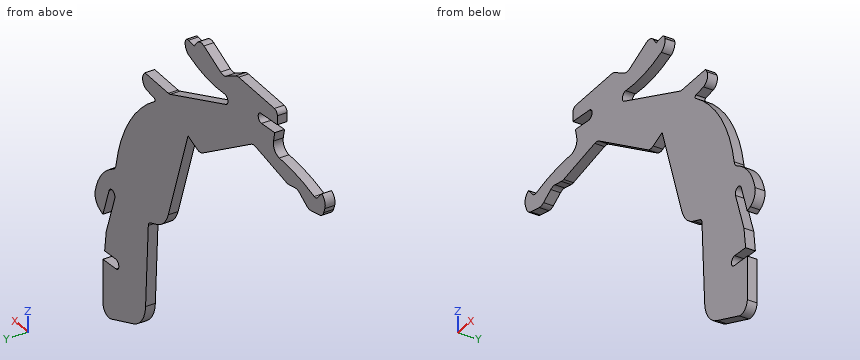
```python
from build123d import *

# Parameters (mm, degrees)
BOSS_EXTRUDE1_DEPTH = 3
FILLET1_R           = 3
FILLET2_R           = 1.5
FILLET3_R           = 10
FILLET4_R           = 3
FILLET5_R           = 4
FILLET6_R           = 2.5
FILLET7_R           = 0.5


with BuildPart() as part:
    # Sketch3 → Boss-Extrude1 (new body)
    with BuildSketch(Plane(origin=(0, 0, 0), x_dir=(1, 0, 0), z_dir=(0, 1, 0))):
        with BuildLine():
            Line((7.923093171, 8.181542538), (1.28839884, 7.442154357))
            Line((1.28839884, 7.442154357), (2.76822933, 14.19))
            ThreePointArc((2.76822933, 14.19), (-8.413807268, 14.494015924), (-19.359710867, 16.8))
            Line((-19.359710867, 16.8), (-22.216794933, 13.666296862))
            Line((-22.216794933, 13.666296862), (-24.820279869, 14.62298821))
            Line((-24.820279869, 14.62298821), (-22.646481841, 20.53863742))
            Line((-22.646481841, 20.53863742), (-15.703804617, 22.111794774))
            Line((-15.703804617, 22.111794774), (-10.073302156, 18.818482014))
            Line((-10.073302156, 18.818482014), (-5.186450964, 19.880840969))
            Line((-5.186450964, 19.880840969), (12.13, 16.8))
            Line((12.13, 16.8), (38.76, 34.29))
            Line((38.76, 34.29), (44.7, 32))
            Line((44.7, 32), (56.058554748, 66.4069852))
            Line((56.058554748, 66.4069852), (64.552315124, 69.756868371))
            Line((64.552315124, 69.756868371), (66.29, 103.00790875))
            Line((66.29, 103.00790875), (87.31, 111.63))
            Line((87.31, 111.63), (87.31, 93.591357519))
            Line((87.31, 93.591357519), (80.722672152, 93.01504101))
            ThreePointArc((80.722672152, 93.01504101), (79.359113719, 91.390015348), (80.984139381, 90.026456915))
            Line((80.984139381, 90.026456915), (86.46321022, 90.505813501))
            Line((86.46321022, 90.505813501), (85.632866314, 84))
            Line((85.632866314, 84), (81.389705108, 71.508585308))
            ThreePointArc((81.389705108, 71.508585308), (82.327545423, 69.605835839), (84.230294892, 70.543676154))
            Line((84.230294892, 70.543676154), (87.31, 79.61))
            Line((87.31, 79.61), (91.618486592, 77.887634392))
            ThreePointArc((91.618486592, 77.887634392), (88.600013238, 68.48894743), (80.984139381, 62.208424889))
            ThreePointArc((80.984139381, 62.208424889), (74.158506271, 43.709858628), (60.297831214, 29.686025056))
            Line((60.297831214, 29.686025056), (68.03871852, 28.66301442))
            ThreePointArc((68.03871852, 28.66301442), (67.586257486, 26.243028794), (66.29, 24.15))
            Line((66.29, 24.15), (54.05, 24.15))
            Line((54.05, 24.15), (25.830040494, 11.99))
            ThreePointArc((25.830040494, 11.99), (24.800734775, 10.253880031), (26.431506195, 9.064692331))
            ThreePointArc((26.431506195, 9.064692331), (36.664028635, 8.803570476), (46.46571567, 5.854056721))
            Line((46.46571567, 5.854056721), (45.9, 1.991540554))
            Line((45.9, 1.991540554), (41.660045255, 2.482673431))
            Line((41.660045255, 2.482673431), (38.9, -1.2))
            Line((38.9, -1.2), (27.015518097, 3.924692331))
            Line((27.015518097, 3.924692331), (20.16, 0))
            Line((20.16, 0), (0, 0))
            Line((0, 0), (0, 4.28))
            Line((0, 4.28), (8.255364291, 5.2))
            ThreePointArc((8.255364291, 5.2), (9.58, 6.856906829), (7.923093171, 8.181542538))
        make_face()
    extrude(amount=BOSS_EXTRUDE1_DEPTH)

    # Fillet1
    # the kernel refuses this fillet: 3 mm, written as the material it adds along each edge
    with BuildSketch(Plane(origin=(80.984139381, 0, -62.208424889), x_dir=(0.9022478681487618, 0, -0.4312177923289046), z_dir=(0, 1, 0))) as fillet1_piece_1:
        with BuildLine():
            CenterArc((1.578679862, -2.997421373), FILLET1_R, 92.37575888, 52.157589609)
            ThreePointArc((-0.864680258, -1.256734347), (-0.427200708, -0.631903288), (0, 0))
            ThreePointArc((0, 0), (0.72716053, -0.015077949), (1.45432106, 0))
        make_face()
    extrude(amount=3)
    with BuildSketch(Plane(origin=(27.015518097, 0, -3.924692331), x_dir=(0.9182659150547935, 0, 0.39596427774305953), z_dir=(0, 1, 0))) as fillet1_piece_2:
        with BuildLine():
            CenterArc((FILLET1_R * 0.49985366711, -FILLET1_R), FILLET1_R, 90, 53.116686758)
            Line((-FILLET1_R * 0.300005823165, -FILLET1_R * 0.399812699386), (0, 0))
            Line((0, 0), (FILLET1_R * 0.49985366711, 0))
        make_face()
    extrude(amount=3)
    with BuildSketch(Plane(origin=(12.13, 0, -16.8), x_dir=(-0.9845393680489544, 0, -0.17516344584919966), z_dir=(0, 1, 0))) as fillet1_piece_3:
        with BuildLine():
            CenterArc((FILLET1_R * 0.397788634748, -FILLET1_R), FILLET1_R, 90, 43.384200988)
            Line((-FILLET1_R * 0.289098500769, -FILLET1_R * 0.273235895863), (0, 0))
            Line((0, 0), (FILLET1_R * 0.397788634748, 0))
        make_face()
    extrude(amount=3)
    with BuildSketch(Plane(origin=(-10.073302156, 0, -18.818482014), x_dir=(-0.863187603129405, 0, -0.5048833150379528), z_dir=(0, 1, 0))) as fillet1_piece_4:
        with BuildLine():
            CenterArc((FILLET1_R * 0.389766900576, -FILLET1_R), FILLET1_R, 90, 42.58838059)
            Line((-FILLET1_R * 0.286959776942, -FILLET1_R * 0.263765659633), (0, 0))
            Line((0, 0), (FILLET1_R * 0.389766900576, 0))
        make_face()
    extrude(amount=3)
    with BuildSketch(Plane(origin=(2.76822933, 0, -14.19), x_dir=(-0.21421340809022724, 0, 0.9767868835085624), z_dir=(0, 1, 0))) as fillet1_piece_5:
        with BuildLine():
            CenterArc((3.855271405, -3), FILLET1_R, 90, 102.505548925)
            ThreePointArc((0.926446282, -3.649602493), (0.490902504, -1.81777488), (0, 0))
            Line((0, 0), (3.855271405, 0))
        make_face()
    extrude(amount=3)
    # the kernel refuses this fillet: 3 mm, written as the material it takes off along each edge
    with BuildSketch(Plane(origin=(-24.820279869, -7.478630688, -14.62298821), x_dir=(0.9386336815677853, 0, 0.3449156590044952), z_dir=(0, 1, 0))) as fillet1_2_piece_1:
        with BuildLine():
            CenterArc((3, 2.991452275), FILLET1_R, 180, 85.673811508)
            Line((0, 2.991452275), (0, 0))
            Line((0, 0), (2.773696477, 0))
        make_face()
    extrude(amount=17.957261376, mode=Mode.SUBTRACT)
    with BuildSketch(Plane(origin=(20.16, -1.994934097, 0), x_dir=(0.8678473261649016, 0, -0.4968309757537575), z_dir=(0, 1, 0))) as fillet1_2_piece_2:
        with BuildLine():
            CenterArc((FILLET1_R * 0.265991212876, FILLET1_R), FILLET1_R, 240.209440415, 29.790559585)
            Line((-FILLET1_R * 0.230839762878, FILLET1_R * 0.132152673835), (0, 0))
            Line((0, 0), (FILLET1_R * 0.265991212876, 0))
        make_face()
    extrude(amount=6.989868193, mode=Mode.SUBTRACT)
    with BuildSketch(Plane(origin=(46.46571567, -6.070952348, -5.854056721), x_dir=(-0.9233291277987619, 0, -0.38400953342121286), z_dir=(0, 1, 0))) as fillet1_2_piece_3:
        with BuildLine():
            CenterArc((2.333722575, 2.99850626), FILLET1_R, 194.249797413, 77.558344276)
            Line((-0.573972765, 2.260056662), (0, 0))
            ThreePointArc((0, 0), (1.21419047, -0.019160317), (2.428380939, 0))
        make_face()
    extrude(amount=15.141904695, mode=Mode.SUBTRACT)
    with BuildSketch(Plane(origin=(38.9, -5.909950036, 1.2), x_dir=(0.5997274231965581, 0, -0.8002043600643629), z_dir=(0, 1, 0))) as fillet1_2_piece_4:
        with BuildLine():
            CenterArc((FILLET1_R * 0.78799333809, FILLET1_R), FILLET1_R, 193.524251091, 76.475748909)
            Line((-FILLET1_R * 0.184277686804, FILLET1_R * 0.766143090435), (0, 0))
            Line((0, 0), (FILLET1_R * 0.78799333809, 0))
        make_face()
    extrude(amount=14.819900071, mode=Mode.SUBTRACT)
    with BuildSketch(Plane(origin=(38.76, -3.852720436, -34.29), x_dir=(-0.8358453893738872, 0, 0.5489649215226915), z_dir=(0, 1, 0))) as fillet1_2_piece_5:
        with BuildLine():
            CenterArc((FILLET1_R * 0.513696058133, FILLET1_R), FILLET1_R, 215.621225969, 54.378774031)
            Line((-FILLET1_R * 0.299188992069, FILLET1_R * 0.417575846005), (0, 0))
            Line((0, 0), (FILLET1_R * 0.513696058133, 0))
        make_face()
    extrude(amount=10.705440872, mode=Mode.SUBTRACT)
    with BuildSketch(Plane(origin=(-5.186450964, -1.481839662, -19.880840969), x_dir=(-0.9771763639228005, 0, 0.2124296443310458), z_dir=(0, 1, 0))) as fillet1_2_piece_6:
        with BuildLine():
            CenterArc((FILLET1_R * 0.197578621542, FILLET1_R), FILLET1_R, 247.647056489, 22.352943511)
            Line((-FILLET1_R * 0.18273230535, FILLET1_R * 0.0751413086926), (0, 0))
            Line((0, 0), (FILLET1_R * 0.197578621542, 0))
        make_face()
    extrude(amount=5.963679323, mode=Mode.SUBTRACT)
    with BuildSketch(Plane(origin=(-15.703804617, -2.961195523, -22.111794774), x_dir=(-0.975276058531981, 0, 0.22099006686800218), z_dir=(0, 1, 0))) as fillet1_2_piece_7:
        with BuildLine():
            CenterArc((FILLET1_R * 0.394826069747, FILLET1_R), FILLET1_R, 226.909202107, 43.090797893)
            Line((-FILLET1_R * 0.288330425897, FILLET1_R * 0.269727994197), (0, 0))
            Line((0, 0), (FILLET1_R * 0.394826069747, 0))
        make_face()
    extrude(amount=8.922391046, mode=Mode.SUBTRACT)
    with BuildSketch(Plane(origin=(-22.646481841, -4.076928403, -20.53863742), x_dir=(-0.3449156590044966, 0, 0.9386336815677849), z_dir=(0, 1, 0))) as fillet1_2_piece_8:
        with BuildLine():
            CenterArc((FILLET1_R * 0.543590453695, FILLET1_R), FILLET1_R, 212.943838396, 57.056161604)
            Line((-FILLET1_R * 0.295613569123, FILLET1_R * 0.456183295506), (0, 0))
            Line((0, 0), (FILLET1_R * 0.543590453695, 0))
        make_face()
    extrude(amount=11.153856805, mode=Mode.SUBTRACT)

    # Fillet2
    fillet2_edges = [part.edges().sort_by_distance(p)[0] for p in [
        (-19.359710867, 1.5, -16.8),
        (64.552315124, 1.5, -69.756868371),
        (45.9, 1.5, -1.991540554),
        (0, 1.5, 0),
    ]]
    fillet(fillet2_edges, radius=FILLET2_R)

    # Fillet3
    fillet3_edges = [part.edges().sort_by_distance(p)[0] for p in [
        (56.058554748, 1.5, -66.4069852),
        (66.29, 1.5, -103.00790875),
    ]]
    fillet(fillet3_edges, radius=FILLET3_R)

    # Fillet4
    fillet4_edges = [part.edges().sort_by_distance(p)[0] for p in [
        (87.31, 1.5, -111.63),
    ]]
    fillet(fillet4_edges, radius=FILLET4_R)

    # Fillet5
    fillet5_edges = [part.edges().sort_by_distance(p)[0] for p in [
        (91.618486592, 1.5, -77.887634392),
    ]]
    fillet(fillet5_edges, radius=FILLET5_R)

    # Fillet6
    fillet6_edges = [part.edges().sort_by_distance(p)[0] for p in [
        (68.03871852, 1.5, -28.66301442),
        (54.05, 1.5, -24.15),
    ]]
    fillet(fillet6_edges, radius=FILLET6_R)

    # Fillet7
    fillet7_edges = [part.edges().sort_by_distance(p)[0] for p in [
        (60.297831214, 1.5, -29.686025056),
    ]]
    fillet(fillet7_edges, radius=FILLET7_R)


solid = part.part
```
Can you work these out from the model? Positions are in its coordinate system, mm. Coordinates: 2 decimals unless noted, no trailing zeros. Loops run counter-clockwise (first coordinate to the right, second up) from the corner with the lowest first, then second, coordinate; pieces in that order, holes last. Notation, with made-up numbers: (82.25, -3) -> (87.25, -3) arc R10 cw to (87.25, 15) -> close; hole circle Ø8 at (7, 80.5). An arc over 180 degrees is marked (long way). Put each result on its own line as item: value. Start each with the question number.
Q1. I'm going to push a flat-ended pin straight in: P1, Ø0.8, axis at y = 1, z = -3, coming from the -X side. Where does the tip first touch, or does it pass through?
Q2. If I drill on line 1 (Z direction, x = 61.5, y = 2.55); line 2 (Z direction, x = 63, y = 0.55); line 3 (X direction, y = 1.3, z = -78.5), over which ranges is the centre line in solid material (lowest first)? Write a range as [from, to].
Q3. I want a section at A-A (x = 16.5). Write out the boundary of the cut face in (y, z).
Q4. I want a section at B-B (z = -99). Write out the boundary of the cut face in (x, y), plus the area to 3 significant figures.
Taken from the geometry:
1. P1: stops at x = 0
2. line 1: z = [-68.55, -30.5], [-29.54, -24.15]
2. line 2: z = [-69.14, -31.59], [-29.33, -24.15]
2. line 3: x = [65.01, 83.76], [86.93, 89.7]
3. outline: (0, -19.67) -> (3, -19.67) -> (3, 0) -> (0, 0) -> close
4. outline: (66.36, 0) -> (87.31, 0) -> (87.31, 3) -> (66.36, 3) -> close
4. area: 62.9 mm2
